The model under review builds one solid part; all positions refer to its coordinate system, in mm. Face numbers are marked on the shaded views. Coordinates: 2 decimals unless noted, no trailing zeros. Order: outer loops, then holes, each group sorted by start corner. A loop starts at its lowest first (then second) coordinate and runs counter-clockwise, first axis right, second up. Notation, with made-up numbers: (68.5, 52.5) - (89.5, 52.5) arc R25 ccw to (89.5, 77.5) - close; hole circle Ø4 at (58.25, 74). An arc over 180 degrees is marked (long way). Answer in a Markdown table with one row per item.
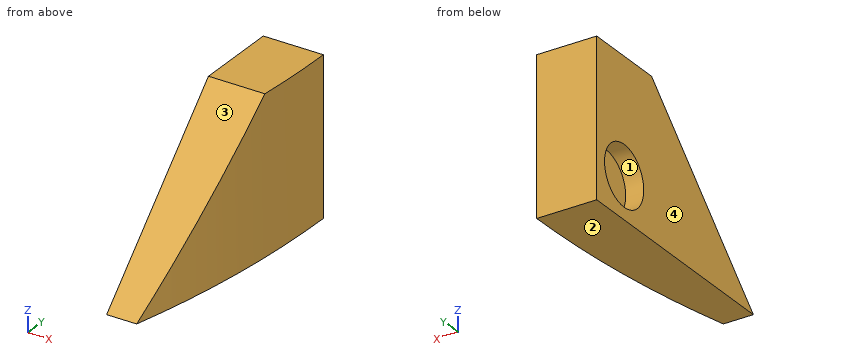
```python
from build123d import *

# Parameters (mm, degrees)
F0_R     = 6.35
F1_DEPTH = 12.7
F2_DEPTH = 3.81
F4_DEPTH = 50.8


with BuildPart() as f1:
    # F0 (on Right) → F1 (new body)
    with BuildSketch(Plane.YZ):
        Polygon((-37.380086, 54.002845), (-70.400086, 20.982845), (-19.600086, 20.982845), (-19.600086, 54.002845), align=None)
        with Locations((-28.490086, 29.872845)):
            Circle(F0_R, mode=Mode.SUBTRACT)
        with Locations((-28.490086, 29.872845)):
            Circle(F0_R)
    extrude(amount=F1_DEPTH)

    # F0 (on Right) → F2 (cut)
    with BuildSketch(Plane.YZ):
        with Locations((-28.490086, 29.872845)):
            Circle(F0_R)
    extrude(amount=F2_DEPTH, mode=Mode.SUBTRACT)

    # F3 (on face) → F4 (cut)
    with BuildSketch(Plane(origin=(0, 0, 20.982845), x_dir=(1, 0, 0), z_dir=(0, 0, -1))):
        with BuildLine():
            ThreePointArc((6.35, 70.400086), (11.106347, 45.197754), (12.7, 19.600086))
            Line((12.7, 19.600086), (12.7, 70.400086))
            Line((12.7, 70.400086), (6.35, 70.400086))
        make_face()
    extrude(amount=-F4_DEPTH, mode=Mode.SUBTRACT)


solid = f1.part
```
Item 1: We need section C-C, the plane x = 2. Write out the cut boundary in (y, z), then the cut area to 3 significant figures.
Check values:
| item | result |
|---|---|
| outline | (-70.4, 20.98) - (-19.6, 20.98) - (-19.6, 54) - (-37.38, 54) - close; hole circle Ø12.7 at (-28.49, 29.87) |
| area | 1,010 mm^2 |
Item 2: We need section B-B, the plane y = -34. Write out the cut boundary in (x, z), then the cut area to 3 significant figures.
Check values:
| item | result |
|---|---|
| outline | (0, 20.98) - (12.2, 20.98) - (12.2, 54) - (0, 54) - (0, 33.03) - (3.81, 33.03) - (3.81, 26.72) - (0, 26.72) - close |
| area | 379 mm^2 |
Item 3: We need section D-D, the plane x = 4.75. Write out the cut boundary in (y, z).
Check values:
| item | result |
|---|---|
| outline | (-70.4, 20.98) - (-19.6, 20.98) - (-19.6, 54) - (-37.38, 54) - close |
Item 4: To check wall thickness, follow line 1 (Z direction, x = 3, y = -27.5); line 2 (Y direction, x = 1.75, z = 25.5); line 3 (Y direction, x = 1.5, z = 35.5). State the ranges of each line that lie inside material, in increasing order. Write a range as from..to.
Check values:
| item | result |
|---|---|
| line 1 | 20.98..23.6, 36.15..54 |
| line 2 | -65.88..-33.09, -23.89..-19.6 |
| line 3 | -55.88..-31.43, -25.55..-19.6 |
Item 5: We need section A-A, the plane z = 32.5. Write out the cut boundary in (x, y), then the cut area to 3 significant figures.
Check values:
| item | result |
|---|---|
| outline | (0, -58.88) - (8.93, -58.88) arc R206.37 ccw to (12.7, -19.6) - (0, -19.6) - (0, -22.71) - (3.81, -22.71) - (3.81, -34.27) - (0, -34.27) - close |
| area | 406 mm^2 |
Item 6: Mouldability with a two-part tool opening along Z and no side actions: class the marked faces 1, 2, 3 and 4 as +Z half, -Z half, draft (parallel to the pull), parting line (faces both ways), or undercut.
Check values:
| item | result |
|---|---|
| face 1 | undercut |
| face 2 | -Z half |
| face 3 | +Z half |
| face 4 | draft |
Item 7: Clearance check with flat-ended pins moving along their axes: pin 1 Ø6 at (x, z) = (6, 34.5) entering from -Y; pin 2 Ø10 at (y, z) = (-27.5, 33) entering from +X; pin 3 Ø7.5 at (y, z) = (-28.49, 29.87) entering from +X. State where each tip first meets the part, or that it passes through.
Check values:
| item | result |
|---|---|
| pin 1 | y = -59.88 |
| pin 2 | x = 12.68 |
| pin 3 | x = 12.64 |
